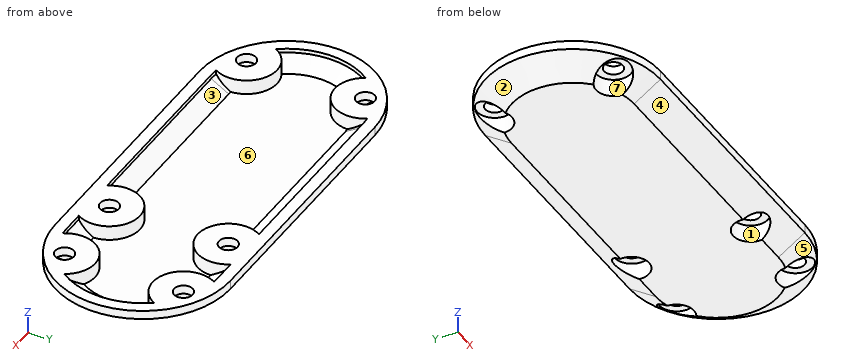
```python
from build123d import *
from OCP.BRepFilletAPI import BRepFilletAPI_MakeChamfer

# Parameters (mm, degrees)
BOSS_EXTRUDE1_DEPTH = 4.5
CUT_EXTRUDE1_DEPTH  = 2.5
CHAMFER1_SIZE       = 1.8
CHAMFER1_SIZE2      = 3
CHAMFER2_SIZE       = 4.5
CHAMFER2_SIZE2      = 3
BOSS_EXTRUDE2_REACH = 56.197
SKETCH3_R           = 2.975
CUT_EXTRUDE2_DEPTH  = 3
CUT_EXTRUDE3_REACH  = 56.093
SKETCH5_R           = 1.6


with BuildPart() as part:
    # Sketch1 → Boss-Extrude1 (new body)
    with BuildSketch(Plane.XY):
        with BuildLine():
            Line((-36.885, 15), (8.115, 15))
            ThreePointArc((8.115, 15), (23.115, 0), (8.115, -15))
            Line((8.115, -15), (-36.885, -15))
            ThreePointArc((-36.885, -15), (-51.885, 0), (-36.885, 15))
        make_face()
    extrude(amount=BOSS_EXTRUDE1_DEPTH)

    # Sketch2 → Cut-Extrude1 (cut)
    with BuildSketch(Plane.XY.offset(4.5)):
        with BuildLine():
            Line((-36.885, 13), (8.115, 13))
            ThreePointArc((8.115, 13), (21.115, 0), (8.115, -13))
            Line((8.115, -13), (-36.885, -13))
            ThreePointArc((-36.885, -13), (-49.885, 0), (-36.885, 13))
        make_face()
    extrude(amount=-CUT_EXTRUDE1_DEPTH, mode=Mode.SUBTRACT)

    # Chamfer1: one chamfer whose edges measure the first distance from different faces: ONE call of the kernel's chamfer builder (chamfer() names one face for all edges)
    chamfer1_edges_1 = [part.edges().sort_by_distance(p)[0] for p in [
        (-49.885, 0, 2),
    ]]
    chamfer1_side_1 = [part.faces().sort_by_distance(p)[0] for p in [
        (-49.885, 0, 3.25),
    ]]
    chamfer1_edges_2 = [part.edges().sort_by_distance(p)[0] for p in [
        (-14.385, 13, 2),
    ]]
    chamfer1_side_2 = [part.faces().sort_by_distance(p)[0] for p in [
        (-14.385, 13, 3.25),
    ]]
    chamfer1_edges_3 = [part.edges().sort_by_distance(p)[0] for p in [
        (21.115, 0, 2),
    ]]
    chamfer1_side_3 = [part.faces().sort_by_distance(p)[0] for p in [
        (21.115, 0, 3.25),
    ]]
    chamfer1_edges_4 = [part.edges().sort_by_distance(p)[0] for p in [
        (-14.385, -13, 2),
    ]]
    chamfer1_side_4 = [part.faces().sort_by_distance(p)[0] for p in [
        (-14.385, -13, 3.25),
    ]]
    chamfer1 = BRepFilletAPI_MakeChamfer(part.part.solid().wrapped)
    for e in chamfer1_edges_1:
        chamfer1.Add(CHAMFER1_SIZE, CHAMFER1_SIZE2, e.wrapped, chamfer1_side_1[0].wrapped)  # the first distance lies on this face
    for e in chamfer1_edges_2:
        chamfer1.Add(CHAMFER1_SIZE, CHAMFER1_SIZE2, e.wrapped, chamfer1_side_2[0].wrapped)  # the first distance lies on this face
    for e in chamfer1_edges_3:
        chamfer1.Add(CHAMFER1_SIZE, CHAMFER1_SIZE2, e.wrapped, chamfer1_side_3[0].wrapped)  # the first distance lies on this face
    for e in chamfer1_edges_4:
        chamfer1.Add(CHAMFER1_SIZE, CHAMFER1_SIZE2, e.wrapped, chamfer1_side_4[0].wrapped)  # the first distance lies on this face
    add(Compound.cast(chamfer1.Shape()), mode=Mode.REPLACE)

    # Chamfer2
    chamfer2_edges = [part.edges().sort_by_distance(p)[0] for p in [
        (-14.385, 15, 0),
        (23.115, 0, 0),
        (-14.385, -15, 0),
        (-51.885, 0, 0),
    ]]
    chamfer2_side = [part.faces().sort_by_distance(p)[0] for p in [
        (-14.385, 0, 0),
    ]]
    chamfer(chamfer2_edges, length=CHAMFER2_SIZE, length2=CHAMFER2_SIZE2, reference=chamfer2_side[0])

    # Sketch4 → Boss-Extrude2 (add, up to next)
    with BuildSketch(Plane.XY.offset(4.5), mode=Mode.PRIVATE) as boss_extrude2_sk1:
        with BuildLine():
            Line((-4.425141241, 13), (4.425141241, 13))
            ThreePointArc((4.425141241, 13), (0, 4.925), (-4.425141241, 13))
        make_face()
    boss_extrude2_tool1 = extrude(boss_extrude2_sk1.sketch, amount=-BOSS_EXTRUDE2_REACH, mode=Mode.PRIVATE) - part.part
    # Sketch4 → Boss-Extrude2 (add, up to next)
    with BuildSketch(Plane.XY.offset(4.5), mode=Mode.PRIVATE) as boss_extrude2_sk2:
        with BuildLine():
            Line((-4.425141241, -13), (4.425141241, -13))
            ThreePointArc((4.425141241, -13), (0, -4.925), (-4.425141241, -13))
        make_face()
    boss_extrude2_tool2 = extrude(boss_extrude2_sk2.sketch, amount=-BOSS_EXTRUDE2_REACH, mode=Mode.PRIVATE) - part.part
    # Sketch4 → Boss-Extrude2 (add, up to next)
    with BuildSketch(Plane.XY.offset(4.5), mode=Mode.PRIVATE) as boss_extrude2_sk3:
        with BuildLine():
            ThreePointArc((-47.376988812, 7.675817271), (-40.134845505, 5.628455832), (-38.287336686, 12.924142208))
            ThreePointArc((-38.287336686, 12.924142208), (-43.38538256, 11.25810937), (-47.376988812, 7.675817271))
        make_face()
    boss_extrude2_tool3 = extrude(boss_extrude2_sk3.sketch, amount=-BOSS_EXTRUDE2_REACH, mode=Mode.PRIVATE) - part.part
    # Sketch4 → Boss-Extrude2 (add, up to next)
    with BuildSketch(Plane.XY.offset(4.5), mode=Mode.PRIVATE) as boss_extrude2_sk4:
        with BuildLine():
            ThreePointArc((9.517336686, 12.924142208), (11.364845505, 5.628455832), (18.606988812, 7.675817271))
            ThreePointArc((18.606988812, 7.675817271), (14.61538256, 11.25810937), (9.517336686, 12.924142208))
        make_face()
    boss_extrude2_tool4 = extrude(boss_extrude2_sk4.sketch, amount=-BOSS_EXTRUDE2_REACH, mode=Mode.PRIVATE) - part.part
    # Sketch4 → Boss-Extrude2 (add, up to next)
    with BuildSketch(Plane.XY.offset(4.5), mode=Mode.PRIVATE) as boss_extrude2_sk5:
        with BuildLine():
            ThreePointArc((18.606988812, -7.675817271), (11.364845505, -5.628455832), (9.517336686, -12.924142208))
            ThreePointArc((9.517336686, -12.924142208), (14.61538256, -11.25810937), (18.606988812, -7.675817271))
        make_face()
    boss_extrude2_tool5 = extrude(boss_extrude2_sk5.sketch, amount=-BOSS_EXTRUDE2_REACH, mode=Mode.PRIVATE) - part.part
    # Sketch4 → Boss-Extrude2 (add, up to next)
    with BuildSketch(Plane.XY.offset(4.5), mode=Mode.PRIVATE) as boss_extrude2_sk6:
        with BuildLine():
            ThreePointArc((-38.287336686, -12.924142208), (-40.134845505, -5.628455832), (-47.376988812, -7.675817271))
            ThreePointArc((-47.376988812, -7.675817271), (-43.38538256, -11.25810937), (-38.287336686, -12.924142208))
        make_face()
    boss_extrude2_tool6 = extrude(boss_extrude2_sk6.sketch, amount=-BOSS_EXTRUDE2_REACH, mode=Mode.PRIVATE) - part.part
    add(boss_extrude2_tool1.solids().sort_by_distance((0, 9.366558, 4.5))[0])
    add(boss_extrude2_tool2.solids().sort_by_distance((0, -9.366558, 4.5))[0])
    add(boss_extrude2_tool3.solids().sort_by_distance((-41.888013, 8.664793, 4.5))[0])
    add(boss_extrude2_tool4.solids().sort_by_distance((13.118013, 8.664793, 4.5))[0])
    add(boss_extrude2_tool5.solids().sort_by_distance((13.118013, -8.664793, 4.5))[0])
    add(boss_extrude2_tool6.solids().sort_by_distance((-41.888013, -8.664793, 4.5))[0])

    # Sketch3 → Cut-Extrude2 (cut)
    with BuildSketch(Plane(origin=(0, 0, 0), x_dir=(-1, 0, 0), z_dir=(0, 0, -1))):
        with Locations((-13.99, 10.175)):
            Circle(SKETCH3_R)
        with Locations((0, 10.175)):
            Circle(SKETCH3_R)
        with Locations((42.76, 10.175)):
            Circle(SKETCH3_R)
        with Locations((42.76, -10.175)):
            Circle(SKETCH3_R)
        with Locations((0, -10.175)):
            Circle(SKETCH3_R)
        with Locations((-13.99, -10.175)):
            Circle(SKETCH3_R)
    extrude(amount=-CUT_EXTRUDE2_DEPTH, mode=Mode.SUBTRACT)

    # Sketch5 → Cut-Extrude3 (cut, up to next)
    with BuildSketch(Plane(origin=(0, 0, 3), x_dir=(-1, 0, 0), z_dir=(0, 0, -1)), mode=Mode.PRIVATE) as cut_extrude3_sk1:
        with Locations((-13.99, 10.175)):
            Circle(SKETCH5_R)
    cut_extrude3_tool1 = extrude(cut_extrude3_sk1.sketch, amount=-CUT_EXTRUDE3_REACH, mode=Mode.PRIVATE) & part.part
    # Sketch5 → Cut-Extrude3 (cut, up to next)
    with BuildSketch(Plane(origin=(0, 0, 3), x_dir=(-1, 0, 0), z_dir=(0, 0, -1)), mode=Mode.PRIVATE) as cut_extrude3_sk2:
        with Locations((0, 10.175)):
            Circle(SKETCH5_R)
    cut_extrude3_tool2 = extrude(cut_extrude3_sk2.sketch, amount=-CUT_EXTRUDE3_REACH, mode=Mode.PRIVATE) & part.part
    # Sketch5 → Cut-Extrude3 (cut, up to next)
    with BuildSketch(Plane(origin=(0, 0, 3), x_dir=(-1, 0, 0), z_dir=(0, 0, -1)), mode=Mode.PRIVATE) as cut_extrude3_sk3:
        with Locations((42.76, 10.175)):
            Circle(SKETCH5_R)
    cut_extrude3_tool3 = extrude(cut_extrude3_sk3.sketch, amount=-CUT_EXTRUDE3_REACH, mode=Mode.PRIVATE) & part.part
    # Sketch5 → Cut-Extrude3 (cut, up to next)
    with BuildSketch(Plane(origin=(0, 0, 3), x_dir=(-1, 0, 0), z_dir=(0, 0, -1)), mode=Mode.PRIVATE) as cut_extrude3_sk4:
        with Locations((42.76, -10.175)):
            Circle(SKETCH5_R)
    cut_extrude3_tool4 = extrude(cut_extrude3_sk4.sketch, amount=-CUT_EXTRUDE3_REACH, mode=Mode.PRIVATE) & part.part
    # Sketch5 → Cut-Extrude3 (cut, up to next)
    with BuildSketch(Plane(origin=(0, 0, 3), x_dir=(-1, 0, 0), z_dir=(0, 0, -1)), mode=Mode.PRIVATE) as cut_extrude3_sk5:
        with Locations((0, -10.175)):
            Circle(SKETCH5_R)
    cut_extrude3_tool5 = extrude(cut_extrude3_sk5.sketch, amount=-CUT_EXTRUDE3_REACH, mode=Mode.PRIVATE) & part.part
    # Sketch5 → Cut-Extrude3 (cut, up to next)
    with BuildSketch(Plane(origin=(0, 0, 3), x_dir=(-1, 0, 0), z_dir=(0, 0, -1)), mode=Mode.PRIVATE) as cut_extrude3_sk6:
        with Locations((-13.99, -10.175)):
            Circle(SKETCH5_R)
    cut_extrude3_tool6 = extrude(cut_extrude3_sk6.sketch, amount=-CUT_EXTRUDE3_REACH, mode=Mode.PRIVATE) & part.part
    add(cut_extrude3_tool1.solids().sort_by_distance((13.99, 10.175, 3))[0], mode=Mode.SUBTRACT)
    add(cut_extrude3_tool2.solids().sort_by_distance((0, 10.175, 3))[0], mode=Mode.SUBTRACT)
    add(cut_extrude3_tool3.solids().sort_by_distance((-42.76, 10.175, 3))[0], mode=Mode.SUBTRACT)
    add(cut_extrude3_tool4.solids().sort_by_distance((-42.76, -10.175, 3))[0], mode=Mode.SUBTRACT)
    add(cut_extrude3_tool5.solids().sort_by_distance((0, -10.175, 3))[0], mode=Mode.SUBTRACT)
    add(cut_extrude3_tool6.solids().sort_by_distance((13.99, -10.175, 3))[0], mode=Mode.SUBTRACT)


solid = part.part
```
Input: part model. Units: mm. Frame: model coordinates. Face numbers are marked on the shaded views. A direction names the side the tool comes from. Give positions to 0.01 mm unless a question says otherwise; leave off trailing zeros. Order: outer loops, then holes, each group sorted by start corner. A loop starts at its lowest first (then second) coordinate and runs counter-clockwise, first axis right, second up.
1. Reachability of the marked faces 5, 6 and 7 from +Z, -Z, +X, -X, +Y, -Y: full face, straight path, thin tool, end or side. Return the list, or none.
Derived:
face 5: -Z, +X
face 6: +Z
face 7: -Z
2. Mould query, pull axis X, two halves, no side actions, for the marked faces 1, 2, 3 and 4. Classes: released by +X, released by -X, zero draft, split by the parting line, or undercut.
Derived:
face 1: undercut
face 2: released by -X
face 3: undercut
face 4: zero draft
3. Pin query (flat end, axial travel): pin 1 (4 mm diameter, centred on x = 0, y = -10.175, fed in from -Z); pin 2 (16 mm diameter, centred on x = -12.5, y = 2.5, fed in from +Z); pin 3 (3 mm diameter, centred on x = 12.5, y = 11.5, fed in from -Z). Return the tip coordinate at first contact, or that it passes through.
Derived:
pin 1: stops at z = 3
pin 2: stops at z = 2.3
pin 3: stops at z = 0.56
4. Material intervals for L1, parallel to Y at x = 13.99, z = 3.75 (3 decimals); L2, parallel to Y at x = -22.5, z = 3.9; L3, parallel to X at y = -8, z = 2.2, sorted ascending.
Derived:
L1: y = -13.802 to -11.775, -8.575 to -4.925, 4.925 to 8.575, 11.775 to 13.802
L2: y = -15 to -13, 13 to 15
L3: x = -48.13 to -44.79, -40.73 to -37.98, -4.78 to -2.03, 2.03 to 4.78, 9.21 to 11.96, 16.02 to 19.36
5. Section C-C on z = 0.85. Return the cut outline in (x, y) (3 decimals).
Derived:
outline: (-45.143, -8.394) arc R2.975 cw to (-40.026, -11.348) arc R11.775 ccw to (-36.885, -11.775) - (-2.508, -11.775) arc R2.975 cw (long way) to (2.508, -11.775) - (8.115, -11.775) arc R11.775 ccw to (11.256, -11.348) arc R2.975 cw to (16.373, -8.394) arc R11.775 ccw to (16.373, 8.394) arc R2.975 cw to (11.256, 11.348) arc R11.775 ccw to (8.115, 11.775) - (2.508, 11.775) arc R2.975 cw (long way) to (-2.508, 11.775) - (-36.885, 11.775) arc R11.775 ccw to (-40.026, 11.348) arc R2.975 cw to (-45.143, 8.394) arc R11.775 ccw to start
6. Section A-A on x = 0. Return the cut outline in (y, z) (3 decimals), and give its area (3 significant figures).
Derived:
outline: (-15, 3) - (-13.15, 1.767) - (-13.15, 3) - (-11.775, 3) - (-11.775, 4.5) - (-15, 4.5) - close; (-8.575, 3) - (-7.2, 3) - (-7.2, 0) - (7.2, 0) - (7.2, 3) - (8.575, 3) - (8.575, 4.5) - (4.925, 4.5) - (4.925, 2) - (-4.925, 2) - (-4.925, 4.5) - (-8.575, 4.5) - close; (11.775, 3) - (13.15, 3) - (13.15, 1.767) - (15, 3) - (15, 4.5) - (11.775, 4.5) - close
area: 56.3 mm2
7. Section B-B on y = 0. Return the cut outline in (x, z) (3 decimals), and give its area (3 significant figures).
Derived:
outline: (-51.885, 3) - (-47.385, 0) - (18.615, 0) - (23.115, 3) - (23.115, 4.5) - (21.115, 4.5) - (21.115, 3.8) - (18.115, 2) - (-46.885, 2) - (-49.885, 3.8) - (-49.885, 4.5) - (-51.885, 4.5) - close
area: 152 mm2
8. Section D-D on x = 13.99. Give the number of separate pieces and of enclosed holes in the cut face, and give its area (3 significant figures).
Derived:
separate pieces: 3
enclosed holes: 0
area: 50.6 mm2
